```python
from build123d import *
from build123d.topology import SkipClean

# Parameters (mm, degrees)
SKETCH_1_R               = 35
EXTRUDE_1_DEPTH          = 3
SKETCH_2_R               = 1.5
CUT_EXTRUDE_1_DEPTH      = 3
SKETCH_3_R               = 1.5
CUT_EXTRUDE_2_DEPTH      = 3
SKETCH_4_R               = 12.5
CUT_EXTRUDE_3_DEPTH      = 3
EXTRUDE_START            = -3
EXTRUDE_4_DEPTH          = 3
FILLET_1_R               = 2
FILLET_2_R               = 2
FILLET_3_R               = 2
FILLET_4_R               = 2
SKETCH_6_R               = 1.5
CUT_EXTRUDE_4_DEPTH      = 3
SKETCH_7_R               = 2
CUT_EXTRUDE_5_DEPTH      = 8
EXTRUDE_7_DEPTH          = 3
SKETCH_10_W              = 42
SKETCH_10_H              = 22
CUT_EXTRUDE_6_DEPTH      = 3
SKETCH_11_R              = 12.5
SKETCH_11_R_2            = 1.5
EXTRUDE_9_DEPTH          = 3
SKETCH_12_W              = 42
SKETCH_12_H              = 22
CUT_EXTRUDE_7_DEPTH      = 3
EXTRUDE_11_DEPTH         = 3
SKETCH_14_R              = 1.5
EXTRUDE_12_DEPTH         = 3
FILLET_5_R               = 2
FILLET_6_R               = 2
FILLET_7_R               = 2
FILLET_8_R               = 2
CUT_EXTRUDE_8_DEPTH      = 57.648036153
CUT_EXTRUDE_8_DEPTH_BACK = 57.648036153
FILLET_9_R               = 1
FILLET_10_R              = 1


with BuildPart() as part:
    # 草图1 → 凸台-拉伸1 (new body)
    with BuildSketch(Plane(origin=(0, 0, 0), x_dir=(0, 0, -1), z_dir=(1, 0, 0))):
        Circle(SKETCH_1_R)
    extrude(amount=EXTRUDE_1_DEPTH)

    # 草图2 → 切除-拉伸1 (cut)
    with BuildSketch(Plane(origin=(3, 0, 0), x_dir=(0, 0, -1), z_dir=(1, 0, 0))):
        with Locations((0, 28)):
            Circle(SKETCH_2_R)
        with Locations((19.798989873, 19.798989873)):
            Circle(SKETCH_2_R)
        with Locations((28, 0)):
            Circle(SKETCH_2_R)
        with Locations((19.798989873, -19.798989873)):
            Circle(SKETCH_2_R)
        with Locations((0, -28)):
            Circle(SKETCH_2_R)
        with Locations((-19.798989873, -19.798989873)):
            Circle(SKETCH_2_R)
        with Locations((-28, 0)):
            Circle(SKETCH_2_R)
        with Locations((-19.798989873, 19.798989873)):
            Circle(SKETCH_2_R)
    extrude(amount=-CUT_EXTRUDE_1_DEPTH, mode=Mode.SUBTRACT)

    # 草图3 → 切除-拉伸2 (cut)
    with BuildSketch(Plane(origin=(3, 0, 0), x_dir=(0, 0, -1), z_dir=(1, 0, 0))):
        with Locations((0, 17.5)):
            Circle(SKETCH_3_R)
        with Locations((12.374368671, 12.374368671)):
            Circle(SKETCH_3_R)
        with Locations((17.5, 0)):
            Circle(SKETCH_3_R)
        with Locations((12.374368671, -12.374368671)):
            Circle(SKETCH_3_R)
        with Locations((0, -17.5)):
            Circle(SKETCH_3_R)
        with Locations((-12.374368671, -12.374368671)):
            Circle(SKETCH_3_R)
        with Locations((-17.5, 0)):
            Circle(SKETCH_3_R)
        with Locations((-12.374368671, 12.374368671)):
            Circle(SKETCH_3_R)
    extrude(amount=-CUT_EXTRUDE_2_DEPTH, mode=Mode.SUBTRACT)

    # 草图4 → 切除-拉伸3 (cut)
    with BuildSketch(Plane.ZY):
        Circle(SKETCH_4_R)
    extrude(amount=-CUT_EXTRUDE_3_DEPTH, mode=Mode.SUBTRACT)

    # 草图5 → 凸台-拉伸4 (add)
    with BuildSketch(Plane(origin=(3, 0, 0), x_dir=(0, 0, -1), z_dir=(1, 0, 0)).offset(EXTRUDE_START)):
        with BuildLine():
            Line((-20, 34.641016151), (-17.5, 30.310889132))
            ThreePointArc((-17.5, 30.310889132), (-9.058666579, 33.80740392), (0, 35))
            Line((0, 35), (0, 40))
            ThreePointArc((0, 40), (-10.352761804, 38.637033052), (-20, 34.641016151))
        make_face()
        with BuildLine():
            ThreePointArc((0, 35), (9.058666579, 33.80740392), (17.5, 30.310889132))
            Line((17.5, 30.310889132), (20, 34.641016151))
            ThreePointArc((20, 34.641016151), (10.352761804, 38.637033052), (0, 40))
            Line((0, 40), (0, 35))
        make_face()
    extrude(amount=EXTRUDE_4_DEPTH)

    # 圆角1
    fillet_1_edges = [part.edges().sort_by_distance(p)[0] for p in [
        (1.5, 34.641016151, 20),
    ]]
    fillet(fillet_1_edges, radius=FILLET_1_R)

    # 圆角2
    fillet_2_edges = [part.edges().sort_by_distance(p)[0] for p in [
        (1.5, 30.310889132, 17.5),
    ]]
    fillet(fillet_2_edges, radius=FILLET_2_R)

    # 圆角3
    fillet_3_edges = [part.edges().sort_by_distance(p)[0] for p in [
        (1.5, 30.310889132, -17.5),
    ]]
    fillet(fillet_3_edges, radius=FILLET_3_R)

    # 圆角4
    fillet_4_edges = [part.edges().sort_by_distance(p)[0] for p in [
        (1.5, 34.641016151, -20),
    ]]
    fillet(fillet_4_edges, radius=FILLET_4_R)

    # 草图6 → 切除-拉伸4 (cut)
    with BuildSketch(Plane(origin=(3, 0, 0), x_dir=(0, 0, -1), z_dir=(1, 0, 0))):
        with Locations((0, 37.5)):
            Circle(SKETCH_6_R)
        with Locations((14.350628714, 34.645482469)):
            Circle(SKETCH_6_R)
        with Locations((-14.350628714, 34.645482469)):
            Circle(SKETCH_6_R)
    extrude(amount=-CUT_EXTRUDE_4_DEPTH, mode=Mode.SUBTRACT)

    # 草图7 → 切除-拉伸5 (cut)
    with BuildSketch(Plane.ZY):
        with Locations((-14.5, 5)):
            Circle(SKETCH_7_R)
        with Locations((-14.5, -5)):
            Circle(SKETCH_7_R)
        with Locations((34.5, -5)):
            Circle(SKETCH_7_R)
        with Locations((34.5, 5)):
            Circle(SKETCH_7_R)
    extrude(amount=-CUT_EXTRUDE_5_DEPTH, mode=Mode.SUBTRACT)

    # 草图8 → 凸台-拉伸7 (add)
    with SkipClean():  # the faces are left unmerged after this step: merging them gives an invalid solid
        with BuildSketch(Plane.ZY):
            with BuildLine():
                Line((37.587704831, 13.680805733), (32.889241728, 11.970705016))
                ThreePointArc((32.889241728, 11.970705016), (33.684327683, 9.506106909), (34.295004854, 6.989466509))
                ThreePointArc((34.295004854, 6.989466509), (35.839777912, 6.484922606), (36.5, 5))
                ThreePointArc((36.5, 5), (36.038906483, 3.722593707), (34.868233163, 3.034191175))
                ThreePointArc((34.868233163, 3.034191175), (35, 0), (34.868233163, -3.034191175))
                ThreePointArc((34.868233163, -3.034191175), (36.038906483, -3.722593707), (36.5, -5))
                ThreePointArc((36.5, -5), (35.839777912, -6.484922606), (34.295004854, -6.989466509))
                ThreePointArc((34.295004854, -6.989466509), (33.684327683, -9.506106909), (32.889241728, -11.970705016))
                Line((32.889241728, -11.970705016), (37.587704831, -13.680805733))
                ThreePointArc((37.587704831, -13.680805733), (39.39231012, -6.945927107), (40, 0))
                ThreePointArc((40, 0), (39.39231012, 6.945927107), (37.587704831, 13.680805733))
            make_face()
        extrude(amount=-EXTRUDE_7_DEPTH)

    # 草图10 → 切除-拉伸6 (cut)
    with SkipClean():  # the faces are left unmerged after this step: merging them gives an invalid solid
        with BuildSketch(Plane.ZY):
            with Locations((10, 0)):
                Rectangle(SKETCH_10_W, SKETCH_10_H)
        extrude(amount=-CUT_EXTRUDE_6_DEPTH, mode=Mode.SUBTRACT)

    # 草图11 → 凸台-拉伸9 (add)
    with SkipClean():  # the faces are left unmerged after this step: merging them gives an invalid solid
        with BuildSketch(Plane.ZY):
            Circle(SKETCH_11_R)
            with Locations((-17.5, 0)):
                Circle(SKETCH_11_R_2)
        extrude(amount=-EXTRUDE_9_DEPTH)

    # 草图12 → 切除-拉伸7 (cut)
    with SkipClean():  # the faces are left unmerged after this step: merging them gives an invalid solid
        with BuildSketch(Plane.ZY):
            with Locations((10, 0)):
                Rectangle(SKETCH_12_W, SKETCH_12_H)
        extrude(amount=-CUT_EXTRUDE_7_DEPTH, mode=Mode.SUBTRACT)

    # 草图13 → 凸台-拉伸11 (add)
    with SkipClean():  # the faces are left unmerged after this step: merging them gives an invalid solid
        with BuildSketch(Plane.ZY.offset(EXTRUDE_START)):
            with BuildLine():
                ThreePointArc((13.874368671, 12.374368671), (11.553207108, 13.629635052), (11.773443753, 11))
                Line((11.773443753, 11), (12.975293589, 11))
                ThreePointArc((12.975293589, 11), (13.629635052, 11.553207108), (13.874368671, 12.374368671))
            make_face()
            with BuildLine():
                Line((12.975293589, -11), (11.773443753, -11))
                ThreePointArc((11.773443753, -11), (11.553207108, -13.629635052), (13.874368671, -12.374368671))
                ThreePointArc((13.874368671, -12.374368671), (13.629635052, -11.553207108), (12.975293589, -11))
            make_face()
        extrude(amount=EXTRUDE_11_DEPTH)

    # 草图14 → 凸台-拉伸12 (add)
    with SkipClean():  # the faces are left unmerged after this step: merging them gives an invalid solid
        with BuildSketch(Plane.ZY.offset(EXTRUDE_START)):
            with Locations((-12.374368671, 12.374368671)):
                Circle(SKETCH_14_R)
            with Locations((0, 17.5)):
                Circle(SKETCH_14_R)
            with Locations((-12.374368671, -12.374368671)):
                Circle(SKETCH_14_R)
            with Locations((0, -17.5)):
                Circle(SKETCH_14_R)
        extrude(amount=EXTRUDE_12_DEPTH)

    # 圆角5
    fillet_5_edges = [part.edges().sort_by_distance(p)[0] for p in [
        (1.5, 13.680805733, 37.587704831),
    ]]
    fillet(fillet_5_edges, radius=FILLET_5_R)

    # 圆角6
    fillet_6_edges = [part.edges().sort_by_distance(p)[0] for p in [
        (1.5, -11.970705016, 32.889241728),
    ]]
    fillet(fillet_6_edges, radius=FILLET_6_R)

    # 圆角7
    fillet_7_edges = [part.edges().sort_by_distance(p)[0] for p in [
        (1.5, 11.970705016, 32.889241728),
    ]]
    fillet(fillet_7_edges, radius=FILLET_7_R)

    # 圆角8
    fillet_8_edges = [part.edges().sort_by_distance(p)[0] for p in [
        (1.5, -13.680805733, 37.587704831),
    ]]
    fillet(fillet_8_edges, radius=FILLET_8_R)

    # 草图15 → 切除-拉伸8 (cut, two sides: drawn at the far end of the back side and taken through both)
    with SkipClean():  # the faces are left unmerged after this step: merging them gives an invalid solid
        with BuildSketch(Plane.ZY.offset(-CUT_EXTRUDE_8_DEPTH_BACK)):
            with BuildLine():
                ThreePointArc((38.255650602, 11.683543854), (37.259018757, 12.877193403), (35.70855681, 12.996113672))
                ThreePointArc((35.70855681, 12.996113672), (37.422754834, 6.598289219), (38, 0))
                ThreePointArc((38, 0), (37.422754834, -6.598289219), (35.70855681, -12.996113672))
                ThreePointArc((35.70855681, -12.996113672), (37.259018757, -12.877193403), (38.255650602, -11.683543854))
                ThreePointArc((38.255650602, -11.683543854), (39.561509224, -5.906520799), (40, 0))
                ThreePointArc((40, 0), (39.561509224, 5.906520799), (38.255650602, 11.683543854))
            make_face()
        extrude(amount=CUT_EXTRUDE_8_DEPTH + CUT_EXTRUDE_8_DEPTH_BACK, mode=Mode.SUBTRACT)

    # 圆角9
    # the kernel refuses this fillet: 1 mm, written as the material it takes off along each edge
    with BuildSketch(Plane(origin=(5.566068235, 12.996113672, 35.70855681), x_dir=(0, -0.3413769828349391, -0.9399264628631933), z_dir=(-1, 0, 0))) as fillet_9_piece_1:
        with BuildLine():
            CenterArc((1.012831861, 0.999999766), FILLET_9_R, 178.49048731, 91.548723167)
            Line((0.013178896, 1.026342685), (-0.0867864, 1.028976977))
            ThreePointArc((-0.0867864, 1.028976977), (-0.096867816, 0.5144998), (-0.099999978, -6.661e-05))
            Line((-0.099999978, -6.661e-05), (-0.002564992, -0.099967099))
            ThreePointArc((-0.002564992, -0.099967099), (0.052736969, -0.100657535), (1.013584648, -0.099999977))
            Line((1.013584648, -0.099999977), (1.013516213, 0))
        make_face()
    extrude(amount=8.132136469, mode=Mode.SUBTRACT)

    # 圆角10
    # the kernel refuses this fillet: 1 mm, written as the material it takes off along each edge
    with BuildSketch(Plane(origin=(-2.566068235, -12.996113672, 35.70855681), x_dir=(0, 0.9442321213290604, 0.3292805810405803), z_dir=(1, 0, 0))) as fillet_10_piece_1:
        with BuildLine():
            CenterArc((1.012921672, -0.999908795), FILLET_10_R, 89.226161317, 91.548723167)
            Line((0.013013123, -1.013432668), (-0.086977731, -1.014785056))
            ThreePointArc((-0.086977731, -1.014785056), (-0.099972117, -0.054025023), (-0.099991792, 0.001281244))
            Line((-0.099991792, 0.001281244), (-0.001350562, 0.099990879))
            ThreePointArc((-0.001350562, 0.099990879), (0.513213647, 0.103465793), (1.027777856, 0.099990879))
            Line((1.027777856, 0.099990879), (1.026427294, 0))
        make_face()
    extrude(amount=8.132136469, mode=Mode.SUBTRACT)


solid = part.part
```
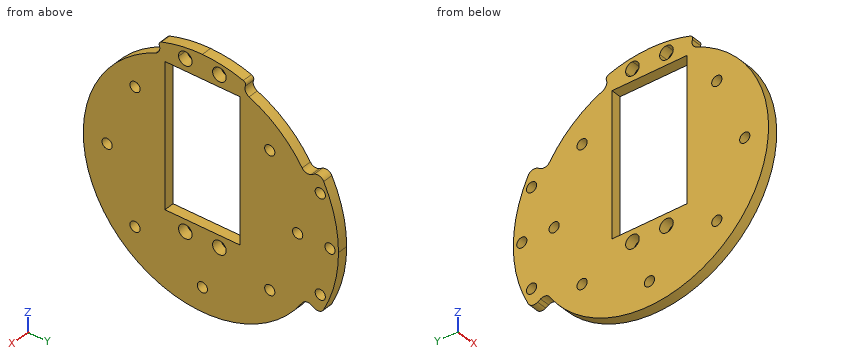
Work out the finished part from the listing and answer in its coordinate system (mm). Round coordinates to 2 decimals unless told otherwise and drop trailing zeros. Write each loop counter-clockwise with the first axis right and the second up, starting at its lowest first coordinate (ties: lowest second). Pieces come first, ordered by that corner, then holes. Notation, with made-up numbers: (-36.5, -4.5) - (-30.5, -4.5) arc R21 ccw to (-30.5, 13.5) - close; hole circle Ø9 at (87, 36). An arc over 180 degrees is marked (long way). Return JSON: item names as keys, results as strings. Group by question number.
Q1. The part is cut by section B-B on y = 25. Write down the section's boundary in (x, z).
Q2. Each of these flat-tipped pins is pushed along its axis until it touches: pin 1 Ø1.5 at (x, z) = (1, 15.5) entering from +Y; pin 2 Ø1 at (x, z) = (0.5, 6) entering from +Y; pin 3 Ø1.5 at (x, y) = (2, -2.5) entering from +Z; pin 4 Ø3 at (y, z) = (-5, -14.5) entering from -X. Where does it stop, or does it pass through?
Q3. The part is cut by section A-A on z = -28. Write down the section's boundary in (x, y).
Q4. Find the intervals of material crossed by L1, parallel to Z at x = 0.55, y = -21; L2, parallel to Z at x = 1.8, y = -1; L3, parallel to Z at x = 1.3, y = 8, in increasing order.
Q5. The part is cut by section D-D on y = -22.5. Write down the section's boundary in (x, z), then the cut area to 3 significant figures.
Q6. The part is cut by section C-C on x = 1.25. Count the separate pieces of the cut face and the enclosed holes in it, then the cut area to 3 significant figures.
Solved:
{
 "1": {"outline": "(0, -24.49) - (3, -24.49) - (3, 24.49) - (0, 24.49) - close"},
 "2": {"pin 1": "y = 37.18", "pin 2": "y = 39.62", "pin 3": "z = 37.96", "pin 4": "through"},
 "3": {"outline": "(0, -21) - (3, -21) - (3, -1.5) - (0, -1.5) - close; (0, 1.5) - (3, 1.5) - (3, 21) - (0, 21) - close"},
 "4": {"L1": "-28 to -20.7, -18.9 to 18.9, 20.7 to 28", "L2": "-34.99 to -29.12, -26.88 to -11, 31 to 37.99", "L3": "-34.07 to -11, 31 to 37.15"},
 "5": {"outline": "(0, -26.81) - (3, -26.81) - (3, 26.81) - (0, 26.81) - close", "area": "161 mm²"},
 "6": {"separate pieces": "1", "enclosed holes": "15", "area": "3,080 mm²"}
}
